from build123d import *

# Parameters (mm, degrees)
F0_R     = 4.35
F4_DEPTH = 3
F5_SIZE  = 0.2


with BuildPart() as f2:
    # F2: sweep along a path in F1
    with BuildLine(Plane.XZ) as f2_path:
        Line((0, 0), (0, 2))
    # F0 (on Top) → F2 (sweep)
    with BuildSketch(Plane.XY):
        with BuildLine():
            Line((1.7, -8.178079), (1.7, -5.178079))
            ThreePointArc((1.7, -5.178079), (0, 5.45), (-1.7, -5.178079))
            Line((-1.7, -5.178079), (-1.7, -8.178079))
            Line((-1.7, -8.178079), (1.7, -8.178079))
        make_face()
        Circle(F0_R, mode=Mode.SUBTRACT)
    sweep(path=f2_path.line)

    # F3 (on face) → F4 (cut)
    with BuildSketch(Plane.XZ.offset(8.178079)):
        with BuildLine():
            Line((-0.6, 2), (-0.6, 1.5))
            ThreePointArc((-0.6, 1.5), (0, 0.9), (0.6, 1.5))
            Line((0.6, 1.5), (0.6, 2))
            Line((0.6, 2), (-0.6, 2))
        make_face()
    extrude(amount=-F4_DEPTH, mode=Mode.SUBTRACT)

    # F5
    f5_edges = [f2.edges().sort_by_distance(p)[0] for p in [
        (-1.7, -6.678079, 0),
        (0, 5.45, 0),
        (0, -8.178079, 0),
        (1.7, -6.678079, 0),
        (-4.35, 0, 0),
    ]]
    chamfer(f5_edges, length=F5_SIZE)


solid = f2.part
Geometry check sheet. Reference: the model listing, model coordinates, mm. A direction names the side the tool comes from. Round coordinates to 2 decimals unless told otherwise and drop trailing zeros. Write each loop counter-clockwise with the first axis right and the second up, starting at its lowest first coordinate (ties: lowest second). Pieces come first, ordered by that corner, then holes. Notation, with made-up numbers: (-22, -18.5) -> (22, -18.5) arc R12 ccw to (22, 1.5) -> close; hole circle Ø6 at (-26, 15). An arc over 180 degrees is marked (long way). One line per item, written item: value. Start each with the question number.
(1) Go/stop test with flat-tipped pins: pin 1 Ø0.6 at (y, z) = (-6.5, 1.5) entering from +X; pin 2 Ø1 at (y, z) = (1, 1) entering from -X. Record where each tip stops, or that it passes through.
(2) Cross-section at A-A, the plane y = 0. Record the cut outline in (x, z), and give its area (3 significant figures).
(3) Access from +Z, -Z, +X, -X, +Y, -Y to the whole of each face (thin tool, end or side, straight path). Record for faces 1 (the flat face through (0, -5.178, 1.5)), 2 (the flat face through (0, -5, 0)), 3 (the flat face through (-1.7, -7, 1)).
(4) Draft check along X on faces 4 (the flat face through (-1.6, -4.4, 2)), 5 (the cylindrical face through (0, -6.7, 0.9)), 6 (the flat face through (1.7, -7, 1)). Enter one of: +X half, -X half, draft (parallel to the pull), parting line (faces both ways), or undercut.
(5) Cross-section at C-C, the plane z = 0.6. Record the cut outline in (x, y).
(6) Cross-section at B-B, the plane x = 0. Record the cut outline in (y, z), and give its area (3 significant figures).
(7) Cross-section at D-D, the plane y = -5.75. Record the cut outline in (x, z).
(8) Scan lines: line 1 (Y direction, x = 0, z = 0.6); line 2 (Y direction, x = 0, z = 1); line 3 (X direction, y = -7.5, z = 1.5). Record each from-to range of solid material in increasing order. Write a range as [from, to].
Answer:
1. pin 1: x = 1.7
1. pin 2: x = -5.43
2. outline: (-5.45, 0.2) -> (-5.25, 0) -> (-4.55, 0) -> (-4.35, 0.2) -> (-4.35, 2) -> (-5.45, 2) -> close; (4.35, 0.2) -> (4.55, 0) -> (5.25, 0) -> (5.45, 0.2) -> (5.45, 2) -> (4.35, 2) -> close
2. area: 4.32 mm²
3. face 1: +Z, -Y
3. face 2: -Z, +X, -X, +Y, -Y
3. face 3: +Z, -Z, -X, -Y
4. face 4: draft
4. face 5: undercut
4. face 6: +X half
5. outline: (-1.7, -8.18) -> (1.7, -8.18) -> (1.7, -5.18) arc R5.45 ccw (long way) to (-1.7, -5.18) -> close; hole circle Ø8.7 at (0, 0)
6. outline: (-8.18, 0.2) -> (-7.98, 0) -> (-4.55, 0) -> (-4.35, 0.2) -> (-4.35, 2) -> (-5.18, 2) -> (-5.18, 0.9) -> (-8.18, 0.9) -> close; (4.35, 0.2) -> (4.55, 0) -> (5.25, 0) -> (5.45, 0.2) -> (5.45, 2) -> (4.35, 2) -> close
6. area: 6.48 mm²
7. outline: (-1.7, 0.2) -> (-1.5, 0) -> (1.5, 0) -> (1.7, 0.2) -> (1.7, 2) -> (0.6, 2) -> (0.6, 1.5) arc R0.6 cw to (-0.6, 1.5) -> (-0.6, 2) -> (-1.7, 2) -> close
8. line 1: [-8.18, -4.35], [4.35, 5.45]
8. line 2: [-5.18, -4.35], [4.35, 5.45]
8. line 3: [-1.7, -0.6], [0.6, 1.7]
